Can you work these out from the model? Positions are in its coordinate system, mm. Give positions to 0.01 mm unless a question says otherwise; leave off trailing zeros. Write each loop counter-clockwise with the first axis right and the second up, starting at its lowest first coordinate (ties: lowest second). Pieces come first, ordered by that corner, then holes.
1. If I drill on probe 1 along Z at (x, y) = (35, -45.5); probe 2 along X at (y, z) = (-65, -68); probe 3 along X at (y, z) = (-75, -44.5), over which ranges is the centre line in solid material (lowest first)?
2. Suppose I cut it at A-A (y = 0). Please give me the cut outline in (x, z), and give its area (3 significant figures).
3. Suppose I cut it at D-D (z = -49). Please give me the cut outline in (x, y).
4. Suppose I cut it at B-B (x = 0). Please give me the cut outline in (y, z) (3 decimals).
5. I'm going to push flat-ended pins straight in: pin 1 (5 mm diameter, centred on x = 0.5, z = -40.5, fed in from +Y); pin 2 (1.5 mm diameter, centred on y = -90, z = -23, fed in from -X); pin 3 (3 mm diameter, centred on y = 49.5, z = -18.5, fed in from -X). Where does each tip first touch, or does it pass through?
6. Suppose I cut it at C-C (z = -64.5). Please give me the cut outline in (x, y), and give its area (3 significant figures).
```python
from build123d import *

# Parameters (mm, degrees)
F3_DEPTH     = 3.175
F4_T1_DEPTH  = 26.7171757075
F4_T3_DEPTH  = 10.7537660931
F4_T5_DEPTH  = 26.7171757075
F4_T8_ANGLE  = 93.1775029202
F4_T10_ANGLE = 82.3499629572
F4_T12_ANGLE = 82.3499629572
F4_T14_ANGLE = 93.1775029202
F4_T16_ANGLE = 8.9450682453


# Not quite as in the source:
# - a fillet or chamfer that OpenCascade refuses, or shapes differently, is made with other operations: its cross-section is extruded or revolved along the edge and cut away or added


with BuildPart() as f1:
    # F0 (on Front) → F1 (revolve)
    with BuildSketch(Plane.XZ):
        with BuildLine():
            Line((126.2178106584, 0), (0, 0))
            Line((0, 0), (0, -75.8794099092))
            Line((0, -75.8794099092), (72.1120906848, -75.8794099092))
            ThreePointArc((72.1120906848, -75.8794099092), (74.7667467473, -75.2978846808), (76.9351825033, -73.6598197328))
            Line((76.9351825033, -73.6598197328), (131.0409024769, -10.4804098236))
            ThreePointArc((131.0409024769, -10.4804098236), (131.98628543, -3.6953439375), (126.2178106584, 0))
        make_face()
    revolve(axis=Axis((0, 0, -37.9397049546), (0, 0, -1)))

    # F2 (on face) → F3 (join)
    with BuildSketch(Plane.XY):
        with BuildLine():
            Line((15.2270092071, -113.3658299561), (11.6703658958, -86.8864461614))
            ThreePointArc((11.6703658958, -86.8864461614), (9.5574744515, -82.9521101243), (5.3768830466, -81.3817707299))
            Line((5.3768830466, -81.3817707299), (0, -81.3817707299))
            Line((0, -81.3817707299), (-5.3768830466, -81.3817707299))
            ThreePointArc((-5.3768830466, -81.3817707299), (-9.5574744515, -82.9521101243), (-11.6703658958, -86.8864461614))
            Line((-11.6703658958, -86.8864461614), (-15.2270092071, -113.3658299561))
            ThreePointArc((-15.2270092071, -113.3658299561), (-13.8726748488, -118.2020582047), (-9.4287069428, -120.5418176958))
            ThreePointArc((-9.4287069428, -120.5418176958), (0, -120.9100092136), (9.4287069428, -120.5418176958))
            ThreePointArc((9.4287069428, -120.5418176958), (13.8726748488, -118.2020582047), (15.2270092071, -113.3658299561))
        make_face()
    extrude(amount=F3_DEPTH)

    # F4: fillet of radius 5.08 on 1 edges, made by hand

    # F4_s2 → F4_t1 (cut)
    with BuildSketch(Plane(origin=(15.2270092071, -113.3658299561, 0), x_dir=(0, 0, 1), z_dir=(-0.1331219793, 0.9910996613, 0))):
        with BuildLine():
            ThreePointArc((0, 0), (2.3071134838, -1.8694797079), (3.175, -4.7092860393))
            Line((3.175, -4.7092860393), (3.175, 0))
            Line((3.175, 0), (0, 0))
        make_face()
    extrude(amount=F4_T1_DEPTH, mode=Mode.SUBTRACT)

    # F4_s4 → F4_t3 (cut)
    with BuildSketch(Plane.YZ.offset(-5.3768830466)):
        with BuildLine():
            ThreePointArc((-81.3817707299, 0), (-83.2512504378, 2.3071134838), (-86.0910567692, 3.175))
            Line((-86.0910567692, 3.175), (-81.3817707299, 3.175))
            Line((-81.3817707299, 3.175), (-81.3817707299, 0))
        make_face()
    extrude(amount=F4_T3_DEPTH, mode=Mode.SUBTRACT)

    # F4_s6 → F4_t5 (cut)
    with BuildSketch(Plane(origin=(-11.6703658958, -86.8864461614, 0), x_dir=(0, 0, 1), z_dir=(-0.1331219793, -0.9910996613, 0))):
        with BuildLine():
            ThreePointArc((0, 0), (2.3071134838, -1.8694797079), (3.175, -4.7092860393))
            Line((3.175, -4.7092860393), (3.175, 0))
            Line((3.175, 0), (0, 0))
        make_face()
    extrude(amount=F4_T5_DEPTH, mode=Mode.SUBTRACT)

    # F4_s7 → F4_t8 (revolve, cut)
    with BuildSketch(Plane(origin=(0, 0, 0), x_dir=(0, 0, 1), z_dir=(-0.9969548301, -0.0779811945, 0))):
        with BuildLine():
            ThreePointArc((0, -120.9100092136), (2.3071134838, -119.0405295057), (3.175, -116.2007231743))
            Line((3.175, -116.2007231743), (3.175, -120.9100092136))
            Line((3.175, -120.9100092136), (0, -120.9100092136))
        make_face()
    revolve(axis=Axis((8.9335263578, -114.2111545246, 3.175), (0, 0, 1)), revolution_arc=F4_T8_ANGLE, mode=Mode.SUBTRACT)

    # F4_s9 → F4_t10 (revolve, cut)
    with BuildSketch(Plane(origin=(11.6703658958, -86.8864461614, 0), x_dir=(0, 0, 1), z_dir=(0.1331219793, -0.9910996613, 0))):
        with BuildLine():
            ThreePointArc((0, 0), (2.3071134838, 1.8694797079), (3.175, 4.7092860393))
            Line((3.175, 4.7092860393), (3.175, 0))
            Line((3.175, 0), (0, 0))
        make_face()
    revolve(axis=Axis((5.3768830466, -87.7317707299, 3.175), (0, 0, 1)), revolution_arc=F4_T10_ANGLE, mode=Mode.SUBTRACT)

    # F4_s11 → F4_t12 (revolve, cut)
    with BuildSketch(Plane.YZ.offset(-5.3768830466)):
        with BuildLine():
            ThreePointArc((-81.3817707299, 0), (-83.2512504378, 2.3071134838), (-86.0910567692, 3.175))
            Line((-86.0910567692, 3.175), (-81.3817707299, 3.175))
            Line((-81.3817707299, 3.175), (-81.3817707299, 0))
        make_face()
    revolve(axis=Axis((-5.3768830466, -87.7317707299, 3.175), (0, 0, 1)), revolution_arc=F4_T12_ANGLE, mode=Mode.SUBTRACT)

    # F4_s13 → F4_t14 (revolve, cut)
    with BuildSketch(Plane(origin=(-15.2270092071, -113.3658299561, 0), x_dir=(0, 0, 1), z_dir=(0.1331219793, 0.9910996613, 0))):
        with BuildLine():
            ThreePointArc((0, 0), (2.3071134838, 1.8694797079), (3.175, 4.7092860393))
            Line((3.175, 4.7092860393), (3.175, 0))
            Line((3.175, 0), (0, 0))
        make_face()
    revolve(axis=Axis((-8.9335263578, -114.2111545246, 3.175), (0, 0, 1)), revolution_arc=F4_T14_ANGLE, mode=Mode.SUBTRACT)

    # F4_s15 → F4_t16 (revolve, cut)
    with BuildSketch(Plane(origin=(0, 0, 0), x_dir=(0, 0, 1), z_dir=(-0.9969548301, 0.0779811945, 0))):
        with BuildLine():
            ThreePointArc((0, -120.9100092136), (2.3071134838, -119.0405295057), (3.175, -116.2007231743))
            Line((3.175, -116.2007231743), (3.175, -120.9100092136))
            Line((3.175, -120.9100092136), (0, -120.9100092136))
        make_face()
    revolve(axis=Axis((0, 0, 3.175), (0, 0, 1)), revolution_arc=F4_T16_ANGLE, mode=Mode.SUBTRACT)


solid = f1.part
```
Checks:
1. probe 1: z = -75.88 to 0
1. probe 2: x = -49.63 to 49.63
1. probe 3: x = -68.99 to 68.99
2. outline: (-131.04, -10.48) - (-76.94, -73.66) arc R6.35 ccw to (-72.11, -75.88) - (72.11, -75.88) arc R6.35 ccw to (76.94, -73.66) - (131.04, -10.48) arc R6.35 ccw to (126.22, 0) - (-126.22, 0) arc R6.35 ccw to start
2. area: 16,200 mm2
3. outline: circle Ø196.11 at (0, 0)
4. outline: (-131.041, -10.48) - (-76.935, -73.66) arc R6.35 ccw to (-72.112, -75.879) - (72.112, -75.879) arc R6.35 ccw to (76.935, -73.66) - (131.041, -10.48) arc R6.35 ccw to (126.218, 0) - (-81.382, 0) arc R5.08 ccw to (-86.091, 3.175) - (-116.201, 3.175) arc R5.08 ccw to (-120.91, 0) - (-126.218, 0) arc R6.35 ccw to start
5. pin 1: stops at y = 107.47
5. pin 2: stops at x = -81.13
5. pin 3: stops at x = -115.42
6. outline: circle Ø169.56 at (0, 0)
6. area: 22,600 mm2
